Verification items for the finished model (mm, model axes). Give positions to 0.01 mm unless a question says otherwise; leave off trailing zeros. Order: outer loops, then holes, each group sorted by start corner. A loop starts at its lowest first (then second) coordinate and runs counter-clockwise, first axis right, second up. Notation, with made-up numbers: M 10,-32.5 L 67,-32.5 A15 cw 67,-28.5 Z; hole C 89.25,62.25 d5. An arc over 180 degrees is marked long. Answer as a JSON object with one key per item and string values.
```python
from build123d import *

# Parameters (mm, degrees)
SCHIZZO1_R                   = 2.1
ESTRUSIONE_ESTRUSIONE1_DEPTH = 3
SMUSSO1_SIZE                 = 2


with BuildPart() as part:
    # Schizzo1 → Estrusione-Estrusione1 (new body)
    with BuildSketch(Plane.XY):
        Polygon((0, 71.847389048), (25, 71.847389048), (25, 12.801854913), (0, 12.801854913), (-25, 12.801854913), (-25, 71.847389048), align=None)
        with Locations((18.75, 57.086005514)):
            Circle(SCHIZZO1_R, mode=Mode.SUBTRACT)
        with Locations((18.75, 27.563238447)):
            Circle(SCHIZZO1_R, mode=Mode.SUBTRACT)
        with Locations(Location((-18.75, 27.563238447, 0), (0, 0, 180))):
            Circle(SCHIZZO1_R, mode=Mode.SUBTRACT)
        with Locations(Location((-18.75, 57.086005514, 0), (0, 0, 180))):
            Circle(SCHIZZO1_R, mode=Mode.SUBTRACT)
        with Locations((0, 58.89473309)):
            Circle(SCHIZZO1_R, mode=Mode.SUBTRACT)
        with Locations((0, 31.80362551)):
            Circle(SCHIZZO1_R, mode=Mode.SUBTRACT)
    extrude(amount=ESTRUSIONE_ESTRUSIONE1_DEPTH)

    # Smusso1
    smusso1_edges = [part.edges().sort_by_distance(p)[0] for p in [
        (-2.1, 58.89473309, 0),
        (-2.1, 31.80362551, 0),
    ]]
    chamfer(smusso1_edges, length=SMUSSO1_SIZE)


solid = part.part
```
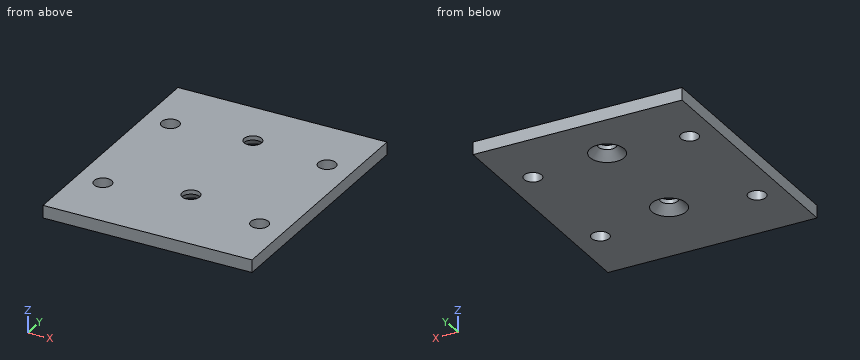
Q1. Section check A-A on x = 0. Record the cut outline in (y, z), then the cut area to 3 significant figures.
Resolved:
{"outline": "M 12.8,0 L 27.7,0 L 29.7,2 L 29.7,3 L 12.8,3 Z; M 33.9,2 L 35.9,0 L 54.79,0 L 56.79,2 L 56.79,3 L 33.9,3 Z; M 60.99,2 L 62.99,0 L 71.85,0 L 71.85,3 L 60.99,3 Z", "area": "144 mm²"}
Q2. Section check C-C on y = 26.5. Record the cut outline in (x, z), then the cut area to 3 significant figures.
Resolved:
{"outline": "M -25,0 L -20.56,0 L -20.56,3 L -25,3 Z; M -16.94,0 L 16.94,0 L 16.94,3 L -16.94,3 Z; M 20.56,0 L 25,0 L 25,3 L 20.56,3 Z", "area": "128 mm²"}
Q3. Gauge pin test, flat ends, axial feed: pin 1 Ø5.5 at (x, y) = (-18.75, 57.09) entering from -Z; pin 2 Ø2.5 at (x, y) = (0, 58.89) entering from -Z; pin 3 Ø6.5 at (x, y) = (0, 31.8) entering from -Z. Record the tip position at first contact, or that the pin passes through.
Resolved:
{"pin 1": "stops at z = 0", "pin 2": "passes through", "pin 3": "stops at z = 0.85"}
Q4. Material ranges on L1, parallel to Y at x = 0, z = 2.3; L2, parallel to Y at x = -18.75, z = 1.8; L3, parallel to X at y = 58.5, z = 1.15, recorded low to high.
Resolved:
{"L1": "y = 12.8 to 29.7, 33.9 to 56.79, 60.99 to 71.85", "L2": "y = 12.8 to 25.46, 29.66 to 54.99, 59.19 to 71.85", "L3": "x = -25 to -20.3, -17.2 to -2.92, 2.92 to 17.2, 20.3 to 25"}
Q5. Section check D-D on x = -18.75. Record the cut outline in (y, z).
Resolved:
{"outline": "M 12.8,0 L 25.46,0 L 25.46,3 L 12.8,3 Z; M 29.66,0 L 54.99,0 L 54.99,3 L 29.66,3 Z; M 59.19,0 L 71.85,0 L 71.85,3 L 59.19,3 Z"}
Q6. Section check B-B on z = 0.65. Record the cut outline in (x, y).
Resolved:
{"outline": "M -25,12.8 L 25,12.8 L 25,71.85 L -25,71.85 Z; hole C -18.75,27.56 d4.2; hole C -18.75,57.09 d4.2; hole C 0,31.8 d6.9; hole C 0,58.89 d6.9; hole C 18.75,27.56 d4.2; hole C 18.75,57.09 d4.2"}
